Geometry: final body of the model. Coordinates: model frame, mm. A direction names the side the tool comes from. Give positions to 0.01 mm unless a question says otherwise; leave off trailing zeros. Order: outer loops, then holes, each group sorted by start corner. A loop starts at its lowest first (then second) coordinate and runs counter-clockwise, first axis right, second up. Notation, with made-up numbers: (87.5, 64) - (94.5, 64) arc R23 cw to (94.5, 80) - close; hole circle Ø4 at (58, 27). An arc over 180 degrees is marked (long way). Use one line per item in the form item = value.
from build123d import *

# Parameters (mm, degrees)
F1_DEPTH       = 32.5
F2_W           = 40
F2_H           = 55
F3_DEPTH       = 60.001
F3_DEPTH_BACK  = 60.001
F4_R           = 5
F6_D           = 5.5
F6_START       = 44.8625
F6_START_2     = 44.8735114
F6_CBORE_D     = 9.75
F6_CBORE_DEPTH = 1
F7_W           = 5
F7_H           = 12
F8_DEPTH       = 0.5358983849
F9_T4_DEPTH    = 13.5430097928
F9_T10_DEPTH   = 13.5430097928


# Not quite as in the source:
# - a fillet or chamfer that OpenCascade refuses, or shapes differently, is made with other operations: its cross-section is extruded or revolved along the edge and cut away or added


with BuildPart() as f1:
    # F0 (on Right) → F1 (new body, symmetric)
    with BuildSketch(Plane.YZ):
        Polygon((0, 50), (0, 60), (-10, 60), (-60, 5), (-60, 0), (60, 0), (60, 5), (15, 50.5358983849), (12, 50.5358983849), (10, 50), align=None)
    extrude(amount=F1_DEPTH, both=True)

    # F2 (on Front) → F3 (cut, two sides)
    with BuildSketch(Plane.XZ) as f3_sk:
        with Locations((0, 32.5)):
            Rectangle(F2_W, F2_H)
    extrude(amount=-F3_DEPTH, mode=Mode.SUBTRACT)
    extrude(f3_sk.sketch, amount=F3_DEPTH_BACK, mode=Mode.SUBTRACT)

    # F4
    f4_edges = [f1.edges().sort_by_distance(p)[0] for p in [
        (20, 0, 5),
        (-20, 0, 5),
    ]]
    fillet(f4_edges, radius=F4_R)

    # F6 (through all)
    # its depths count from where the whole tool has entered the part; down to there all is cleared
    with Locations(Plane.XY.offset(50)):
        with Locations((-26.25, 55, -F6_START_2), (26.25, 55, -F6_START_2), (-26.25, -55, -F6_START), (26.25, -55, -F6_START)):
            CounterBoreHole(F6_D / 2, F6_CBORE_D / 2, F6_CBORE_DEPTH)

    # F7 (on face) → F8 (join, through all)
    with BuildSketch(Plane.XY.offset(50)):
        with Locations((-30, 6)):
            Rectangle(F7_W, F7_H)
        with Locations((30, 6)):
            Rectangle(F7_W, F7_H)
    extrude(amount=F8_DEPTH)

    # F9: chamfer of 0.6 on 2 edges, made by hand


with BuildPart() as f9_tool2:
    # F9_s3 → F9_t4 (new body)
    with BuildSketch(Plane.XZ.offset(-13.5430097928)):
        Polygon((27.5, 49.9358983849), (28.1, 50.5358983849), (27.5, 50.5358983849), align=None)
    extrude(amount=F9_T4_DEPTH)

    split(bisect_by=Plane(origin=(0, -11.8301270189, 44.1506350946), x_dir=(1, 0, 0), z_dir=(0, -0.2588190451, 0.9659258263)), keep=Keep.TOP)

    split(bisect_by=Plane.XY.offset(50), keep=Keep.TOP)


with BuildPart() as f1_1:
    add(f1.part)

    # F9_t1: cut F9_tool2
    add(f9_tool2.part, mode=Mode.SUBTRACT)


with BuildPart() as f9_tool8:
    # F9_s9 → F9_t10 (new body)
    with BuildSketch(Plane.XZ):
        Polygon((-27.5, 49.9358983849), (-28.1, 50.5358983849), (-27.5, 50.5358983849), align=None)
    extrude(amount=-F9_T10_DEPTH)

    split(bisect_by=Plane(origin=(0, -11.8301270189, 44.1506350946), x_dir=(1, 0, 0), z_dir=(0, -0.2588190451, 0.9659258263)), keep=Keep.TOP)

    split(bisect_by=Plane.XY.offset(50), keep=Keep.TOP)


with BuildPart() as f1_2:
    add(f1_1.part)

    # F9_t7: cut F9_tool8
    add(f9_tool8.part, mode=Mode.SUBTRACT)


solid = f1_2.part
(1) Cut plane B-B on y = -18. Output: boundary loops of the cut face in (x, z), plus the area to 3 significant figures.
Computed values:
outline = (-32.5, 0) - (32.5, 0) - (32.5, 51.2) - (20, 51.2) - (20, 10) arc R5 cw to (15, 5) - (-15, 5) arc R5 cw to (-20, 10) - (-20, 51.2) - (-32.5, 51.2) - close
area = 1,490 mm²
(2) Ray query, line 1 along Y through (x, z) = (-26.25, 3.1); line 2 along X through (y, z) = (-55, 9.5) (3 decimals); line 3 along X through (y, z) = (19.5, 12.5). Return the intervals inside material, ascending.
Computed values:
line_1 = -60 to -57.75, -52.25 to 52.25, 57.75 to 60
line_2 = -32.5 to -31.125, -21.375 to -19.975, 19.975 to 21.375, 31.125 to 32.5
line_3 = -32.5 to -20, 20 to 32.5
(3) Reachability of faces 1 (the face through (0, -60, 3)), 2 (the face through (19, 1, 7)), 3 (the face through (-24, 53, 4.126)) from +Z, -Z, +X, -X, +Y, -Y: full face, straight path, thin tool, end or side. Return the list, or none.
Computed values:
face_1 = +Z, -Z, +X, -X, -Y
face_2 = +Z, +Y, -Y
face_3 = +Z
(4) Cut plane D-D on z = 54. Output: boundary loops of the cut face in (x, y).
Computed values:
outline = (-32.5, -15.45) - (-20, -15.45) - (-20, 0) - (-32.5, 0) - close; (20, -15.45) - (32.5, -15.45) - (32.5, 0) - (20, 0) - close
(5) Cut plane C-C on x = -26.25. Give the number of separate pieces and of enclosed holes in the cut face, plus the area to 3 significant figures.
Computed values:
separate_pieces = 3
enclosed_holes = 0
area = 4,060 mm²
(6) Pull-direction query (X, two-part tool) for faces 4 (the face through (-25.572, 32.815, 32.509)), 5 (the face through (-32.5, -1, 23)), 6 (the face through (-25.892, -52.273, 2.04)); classes: released by +X, released by -X, zero draft, split by the parting line, or undercut.
Computed values:
face_4 = zero draft
face_5 = released by -X
face_6 = undercut
(7) Contact query for flat-ended pins moving along their axis: pin 1 Ø11 at (x, y) = (-26.25, -55) entering from +Z; pin 2 Ø5 at (x, y) = (-26.25, -55) entering from -Z; pin 3 Ø6 at (x, y) = (-23, 6) entering from +Z; pin 4 Ø10 at (x, z) = (-19, 53.5) entering from +Y. Output: stop coordinate, or through.
Computed values:
pin_1 = 16.55
pin_2 = through
pin_3 = 50
pin_4 = 16.91
(8) Cut plane A-A on z = 47. Output: boundary loops of the cut face in (x, y).
Computed values:
outline = (-32.5, -21.82) - (-20, -21.82) - (-20, 18.49) - (-32.5, 18.49) - close; (20, -21.82) - (32.5, -21.82) - (32.5, 18.49) - (20, 18.49) - close
